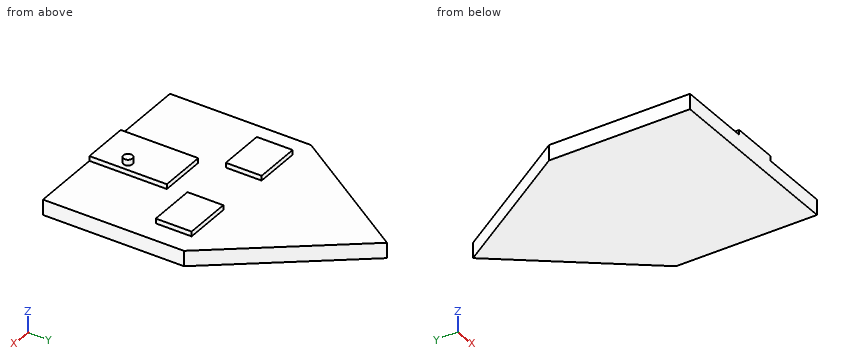
```python
from build123d import *

# Parameters (mm, degrees)
F2_DEPTH  = 5.08
F1_W      = 52.124873735
F1_H      = 98.4580833465
F1_W_2    = 54.0554076433
F1_H_2    = 52.1248690784
F1_W_3    = 53.0901476741
F1_H_3    = 52.1248728037
F3_DEPTH  = 7.62
F4_DEPTH  = 7.62
F5_W      = 62.6767296344
F5_H      = 102.3222543299
F6_DEPTH  = 6.35
F7_R      = 5.9501097349
F8_DEPTH  = 7.62
F9_W      = 61.9803220034
F9_H      = 47.3557561636
F9_W_2    = 63.3731409907
F9_H_2    = 47.3557598889
F10_DEPTH = 6.35


with BuildPart() as f2:
    # F0 (on Top) → F2 (new body)
    with BuildSketch(Plane.XY):
        Polygon((-23.608982563, 281.8368527174), (-140.678524971, 104.0368527174), (-66.4795190096, 104.0368527174), (-61.5329220891, 104.0368527174), (-23.608982563, 104.0368527174), align=None)
        Polygon((113.321475029, 104.0368527174), (-23.608982563, 281.8368527174), (-23.608982563, 104.0368527174), align=None)
        Polygon((-66.4795190096, 104.0368527174), (-140.678524971, 104.0368527174), (-140.678524971, -82.2851061821), (113.321475029, -82.2851061821), (113.321475029, 104.0368527174), (-23.608982563, 104.0368527174), (-61.5329220891, 104.0368527174), align=None)
    extrude(amount=F2_DEPTH)

    # F1 (on face) + F2_face (on face) → F3 (join)
    with BuildSketch(Plane.XY):
        with Locations((-13.7297245674, -28.9409598336)):
            Rectangle(F1_W, F1_H)
        with Locations((58.6659163237, 62.7601984888)):
            Rectangle(F1_W_2, F1_H_2)
        with Locations((-93.3649428189, 57.9338222742)):
            Rectangle(F1_W_3, F1_H_3)
    with BuildSketch(Plane(origin=(-14.7477440157, 60.1118346493, 5.08), x_dir=(1, 0, 0), z_dir=(0, 0, 1))):
        Polygon((-8.8612385473, 221.7250180681), (-125.9307809553, 43.9250180681), (-125.9307809553, -142.3969408314), (128.0692190447, -142.3969408314), (128.0692190447, 43.9250180681), align=None)
    extrude(amount=F3_DEPTH)

    # F1 (on face) + F3_face (on face) → F4 (join)
    with BuildSketch(Plane.XY):
        with Locations((-13.7297245674, -28.9409598336)):
            Rectangle(F1_W, F1_H)
        with Locations((58.6659163237, 62.7601984888)):
            Rectangle(F1_W_2, F1_H_2)
        with Locations((-93.3649428189, 57.9338222742)):
            Rectangle(F1_W_3, F1_H_3)
    with BuildSketch(Plane(origin=(-14.7477440157, 60.1118346493, 12.7), x_dir=(1, 0, 0), z_dir=(0, 0, 1))):
        Polygon((128.0692190447, 43.9250180681), (-8.8612385473, 221.7250180681), (-125.9307809553, 43.9250180681), (-125.9307809553, -142.3969408314), (128.0692190447, -142.3969408314), align=None)
    extrude(amount=F4_DEPTH)

    # F5 (on face) → F6 (join)
    with BuildSketch(Plane.XY.offset(20.32)):
        with Locations((-10.8928931877, -31.1239790171)):
            Rectangle(F5_W, F5_H)
    extrude(amount=F6_DEPTH)

    # F7 (on face) → F8 (join)
    with BuildSketch(Plane.XY.offset(26.67)):
        with Locations((7.9101277515, -39.591267705)):
            Circle(F7_R)
    extrude(amount=F8_DEPTH)

    # F9 (on face) → F10 (join)
    with BuildSketch(Plane.XY.offset(20.32)):
        with Locations((-82.2747275233, 74.1913020611)):
            Rectangle(F9_W, F9_H)
        with Locations((52.8284572065, 71.4056696743)):
            Rectangle(F9_W_2, F9_H_2)
    extrude(amount=F10_DEPTH)


solid = f2.part
```
For this review, take the finished solid that the model builds, in its own axes (mm). Coordinates: 2 decimals unless noted, no trailing zeros. Loops run counter-clockwise (first coordinate to the right, second up) from the corner with the lowest first, then second, coordinate; pieces in that order, holes last. Notation, with made-up numbers: (8, 20) -> (45, 20) arc R24 cw to (45, 39) -> close; hole circle Ø10 at (17.25, -33.75). An arc over 180 degrees is marked (long way). Return JSON: item names as keys, results as strings. Group by question number.
(1) For pin 1 Ø3 at (y, z) = (64.5, 24) entering from +X (3 decimals); pin 2 Ø1 at (x, y) = (28, 113.5) entering from +Z; pin 3 Ø19 at (x, y) = (-13.5, -25) entering from +Z, all flat-tipped, find the tip position at first contact; note any pin that passes through.
(2) Consider section D-D, the plane x = -10.5. Give the boundary of the cut face in (y, z).
(3) Consider section C-C, the plane x = -82. Give the boundary of the cut face in (y, z), plus the area to 3 significant figures.
(4) Consider section A-A, the plane y = 70. Give the boundary of the cut face in (x, z), plus the area to 3 significant figures.
(5) Consider section B-B, the plane z = 4. Give the boundary of the cut face in (x, y), plus the area to 3 significant figures.
(6) To check wall thickness, follow L1, parallel to Z at x = -46.5, y = 19; L2, parallel to Y at x = 64.5, z = 22.5; L3, parallel to Y at x = -98, z = 25.5. State the ranges of each line that lie inside material, in increasing order.
Results below:
{
 "1": {"pin 1": "stops at x = 84.515", "pin 2": "stops at z = 20.32", "pin 3": "stops at z = 26.67"},
 "2": {"outline": "(-82.29, 0) -> (264.82, 0) -> (264.82, 20.32) -> (20.04, 20.32) -> (20.04, 26.67) -> (-82.29, 26.67) -> close"},
 "3": {"outline": "(-82.29, 0) -> (193.16, 0) -> (193.16, 20.32) -> (97.87, 20.32) -> (97.87, 26.67) -> (50.51, 26.67) -> (50.51, 20.32) -> (-82.29, 20.32) -> close", "area": "5,900 mm2"},
 "4": {"outline": "(-140.68, 0) -> (113.32, 0) -> (113.32, 20.32) -> (84.52, 20.32) -> (84.52, 26.67) -> (21.14, 26.67) -> (21.14, 20.32) -> (-51.28, 20.32) -> (-51.28, 26.67) -> (-113.26, 26.67) -> (-113.26, 20.32) -> (-140.68, 20.32) -> close", "area": "5,960 mm2"},
 "5": {"outline": "(-140.68, -82.29) -> (113.32, -82.29) -> (113.32, 104.04) -> (-23.61, 281.84) -> (-140.68, 104.04) -> close", "area": "69,900 mm2"},
 "6": {"L1": "z = 0 to 20.32", "L2": "y = 47.73 to 95.08", "L3": "y = 50.51 to 97.87"}
}
